```python
from build123d import *

# Parameters (mm, degrees)
SKETCH1_W           = 60
SKETCH1_H           = 60
SKETCH1_R           = 3.25
BOSS_EXTRUDE1_DEPTH = 20
CHAMFER1_SIZE       = 2


with BuildPart() as part:
    # Sketch1 → Boss-Extrude1 (new body)
    with BuildSketch(Plane.XY):
        Rectangle(SKETCH1_W, SKETCH1_H)
        with Locations((-15, 20)):
            Circle(SKETCH1_R, mode=Mode.SUBTRACT)
        with Locations((15, 20)):
            Circle(SKETCH1_R, mode=Mode.SUBTRACT)
        with Locations((15, -20)):
            Circle(SKETCH1_R, mode=Mode.SUBTRACT)
        with Locations((-15, -20)):
            Circle(SKETCH1_R, mode=Mode.SUBTRACT)
    extrude(amount=BOSS_EXTRUDE1_DEPTH)

    # Chamfer1
    chamfer1_edges = [part.edges().sort_by_distance(p)[0] for p in [
        (30, -30, 10),
        (-30, -30, 10),
        (-30, 30, 10),
        (30, 30, 10),
    ]]
    chamfer(chamfer1_edges, length=CHAMFER1_SIZE)


solid = part.part
```
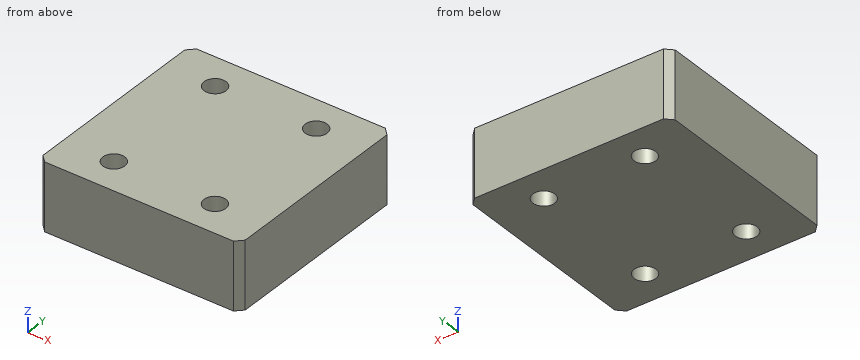
The model under review builds one solid part; all positions refer to its coordinate system, in mm. Round coordinates to 2 decimals unless told otherwise and drop trailing zeros. Loops run counter-clockwise (first coordinate to the right, second up) from the corner with the lowest first, then second, coordinate; pieces in that order, holes last. Notation, with made-up numbers: (29, 41.25) - (56, 41.25) arc R27 ccw to (56, 66.25) - close; hole circle Ø10 at (-1, 69.25). An arc over 180 degrees is marked (long way). Use a Markdown table: item, result. Add a question column.
Q1. Add section A-A (x = 15). State the section outline as (y, z) points.
Q2. Add section B-B (y = -20). State the section outline as (x, z) points.
Q3. Add section C-C (z = 17.5). State the section outline as (x, y) points.
Q4. For probe 1 along Y at (x, z) = (15, 12.5); probe 2 along Y at (x, z) = (-14, 14.5); probe 3 along X at (y, z) = (-21, 10.5), list the stretches that pass through material, from the lowest coordinate up.
Worked answers:
| question | item | result |
|---|---|---|
| 1 | outline | (-30, 0) - (-23.25, 0) - (-23.25, 20) - (-30, 20) - close; (-16.75, 0) - (16.75, 0) - (16.75, 20) - (-16.75, 20) - close; (23.25, 0) - (30, 0) - (30, 20) - (23.25, 20) - close |
| 2 | outline | (-30, 0) - (-18.25, 0) - (-18.25, 20) - (-30, 20) - close; (-11.75, 0) - (11.75, 0) - (11.75, 20) - (-11.75, 20) - close; (18.25, 0) - (30, 0) - (30, 20) - (18.25, 20) - close |
| 3 | outline | (-30, -28) - (-28, -30) - (28, -30) - (30, -28) - (30, 28) - (28, 30) - (-28, 30) - (-30, 28) - close; hole circle Ø6.5 at (-15, -20); hole circle Ø6.5 at (-15, 20); hole circle Ø6.5 at (15, -20); hole circle Ø6.5 at (15, 20) |
| 4 | probe 1 | -30 to -23.25, -16.75 to 16.75, 23.25 to 30 |
| 4 | probe 2 | -30 to -23.09, -16.91 to 16.91, 23.09 to 30 |
| 4 | probe 3 | -30 to -18.09, -11.91 to 11.91, 18.09 to 30 |
